from build123d import *

# Parameters (mm, degrees)
CROQUIS1_W              = 7.7
CROQUIS1_H              = 7.7
SALIENTE_EXTRUIR1_DEPTH = 2.5
CROQUIS2_R              = 1.4
SALIENTE_EXTRUIR2_DEPTH = 3
CROQUIS6_R              = 0.6
CORTAR_EXTRUIR1_DEPTH   = 8.739186004


with BuildPart() as part:
    # Croquis1 → Saliente-Extruir1 (new body)
    with BuildSketch(Plane.XY):
        Rectangle(CROQUIS1_W, CROQUIS1_H)
    extrude(amount=SALIENTE_EXTRUIR1_DEPTH)

    # Croquis2 → Saliente-Extruir2 (add)
    with BuildSketch(Plane(origin=(0, 0, 0), x_dir=(-1, 0, 0), z_dir=(0, 0, -1))):
        Circle(CROQUIS2_R)
    saliente_extruir2 = extrude(amount=SALIENTE_EXTRUIR2_DEPTH)

    # Croquis6 → Cortar-Extruir1 (cut, through all)
    with BuildSketch(Plane(origin=(0, 0, -3), x_dir=(-1, 0, 0), z_dir=(0, 0, -1))):
        Circle(CROQUIS6_R)
    extrude(amount=-CORTAR_EXTRUIR1_DEPTH, mode=Mode.SUBTRACT)

    # Simetría3: Saliente-Extruir2 across plane
    add(saliente_extruir2.mirror(Plane(origin=(0, 0, 1.25), x_dir=(1, 0, 0), z_dir=(0, 0, -1))))


solid = part.part
Here's how the part is built. I have some questions about the finished solid (model axes, mm). A direction names the side the tool comes from. Coordinates: 2 decimals unless noted, no trailing zeros. Order: outer loops, then holes, each group sorted by start corner. A loop starts at its lowest first (then second) coordinate and runs counter-clockwise, first axis right, second up. Notation, with made-up numbers: M 52,35.25 L 88,35.25 A18 cw 88,57.25 Z; hole C 51.25,0.5 d3. An arc over 180 degrees is marked long. Answer as CSV lines item,"result". Start each with the question number.
1. I want a section at B-B, the plane z = 1.5. Write out the boundary of the cut face in (x, y), and give its area (3 significant figures).
2. I want a section at D-D, the plane z = 3.5. Write out the boundary of the cut face in (x, y), and give its area (3 significant figures).
3. I need wall thicknesses on line 1 (Y direction, x = 0, z = -0.7); line 2 (Z direction, x = -3.5, y = 1.25); line 3 (Y direction, x = -1, z = -1). Which ranges of each line are inside material? Lowest first, please. Write a range as [from, to].
4. We'd pull the mould along Y, two halves only. Please class faces 1 (the cylindrical face through (1.4, 0.06, 3.98)), 2 (the flat face through (0, 3.85, 1)), 3 (the flat face through (0, -1, -3)), 4 (the cylindrical face through (-0.323, 0.506, -0.288)): released by +Y, released by -Y, zero draft, split by the parting line, or undercut.
5. On a 3-axis mill with a long thin cutter (end or side, diameter ignored), from which of +Z, -Z, +X, -X, +Y, -Y can I reach the whole of each face in a straight line? I mean faces 5 (the flat face through (0, 0, 2.5)), 6 (the flat face through (-2, 0, 2.5)), 7 (the flat face through (0, 0, 5.5)). Say none if no direction works.
6. For pin 1 (1.5 mm diameter, centred on x = -3, y = -1, fed in from +Z); pin 2 (1.4 mm diameter, centred on x = 0, y = 0, fed in from -Z); pin 3 (2 mm diameter, centred on x = 1, y = -3, fed in from -Z); pin 4 (1 mm diameter, centred on x = -2.5, z = 3.5, fed in from +Y), each with a flat end and sliding along its axis, tell me the tip position at first contact or that it passes through.
7. I want a section at A-A, the plane x = 0. Write out the boundary of the cut face in (y, z).
Recorded:
1,outline,"M -3.85,-3.85 L 3.85,-3.85 L 3.85,3.85 L -3.85,3.85 Z; hole C 0,0 d1.2"
1,area,"58.2 mm2"
2,outline,"C 0,0 d2.8"
2,area,"6.16 mm2"
3,line 1,"y = [-1.4, -0.6], [0.6, 1.4]"
3,line 2,"z = [0, 2.5]"
3,line 3,"y = [-0.98, 0.98]"
4,face 1,"split by the parting line"
4,face 2,"released by +Y"
4,face 3,"zero draft"
4,face 4,"undercut"
5,face 5,"-Z"
5,face 6,"+Z"
5,face 7,"+Z, +X, -X, +Y, -Y"
6,pin 1,"stops at z = 2.5"
6,pin 2,"stops at z = -3"
6,pin 3,"stops at z = 0"
6,pin 4,"passes through"
7,outline,"M -3.85,0 L -1.4,0 L -1.4,-3 L -0.6,-3 L -0.6,2.5 L 0.6,2.5 L 0.6,-3 L 1.4,-3 L 1.4,0 L 3.85,0 L 3.85,2.5 L 1.4,2.5 L 1.4,5.5 L -1.4,5.5 L -1.4,2.5 L -3.85,2.5 Z"
